Autodesk Inventor part; units mm, degrees
ref_plane "YZ Plane" through (0, 0, 0) normal (1, 0, 0) x (0, 1, 0)
ref_plane "XZ Plane" through (0, 0, 0) normal (0, 1, 0) x (-1, 0, 0)
ref_plane "XY Plane" through (0, 0, 0) normal (0, 0, 1) x (1, 0, 0)
sketch "Sketch1" plane through (0, 0, 0) normal (0, 0, 1) x (1, 0, 0)
  line L0 (0, 0) -> (53, 0)
  line L1 (53, 0) -> (53, -50)
  line L2 (53, -50) -> (0, -50)
  line L3 (0, -50) -> (0, 0)
  line L4 (41, 0) -> (41, 6.0159) construction
  line L5 (41, 6.0159) -> (41, -25.0024) construction
  circle A0 centre (41, -5) radius 1.5
  line L6 (41, 3.3654) -> (9, 3.3654) construction
  line L7 (9, 3.3654) -> (9, -23.8563) construction
  line L8 (41, -5) -> (7.1054, -5) construction
  circle A1 centre (9, -5) radius 1.5
  dimension "d0" = 53
  dimension "d1" = 50
  dimension "d2" = 3
  dimension "d3" = 32
  dimension "d4" = 3
extrude "Extrusion1" add sketch "Sketch1" along normal blind 3
sketch "Sketch2" plane through (0, 0, 3) normal (0, 0, 1) x (1, 0, 0)
  line L0 (53, -50) -> (15, -50)
  line L1 (15, -50) -> (15, -47)
  line L2 (15, -47) -> (53, -47)
  line L3 (53, -47) -> (53, -50)
  dimension "d7" = 38
  dimension "d8" = 3
extrude "Extrusion2" add sketch "Sketch2" against normal blind 12
fillet "Fillet3" radius 2 1 edges at (53, -48.5, -9)
fillet "Fillet6" radius 2 1 edges at (15, -48.5, -9)
sketch "Sketch5" plane through (0, 0, 3) normal (0, 0, 1) x (1, 0, 0)
  line L0 (18.1552, -8.3715) -> (42.9873, -8.3715)
  line L1 (42.9873, -8.3715) -> (42.9873, -35.5989)
  line L2 (42.9873, -35.5989) -> (18.1552, -35.5989)
  line L3 (18.1552, -35.5989) -> (18.1552, -8.3715)
extrude "Extrusion4" cut sketch "Sketch5" against normal through all
fillet "Fillet8" radius 2 1 edges at (18.1552, -8.3715, 1.5)
fillet "Fillet9" radius 2 1 edges at (42.9873, -8.3715, 1.5)
fillet "Fillet10" radius 2 1 edges at (18.1552, -35.5989, 1.5)
fillet "Fillet12" radius 2 1 edges at (42.9873, -35.5989, 1.5)
fillet "Fillet13" radius 2 1 edges at (0, 0, 1.5)
fillet "Fillet14" radius 2 1 edges at (53, 0, 1.5)
hole "Hole3" at (17.1081, -4.4429, 3) direction (0, 0, -1) diameter 3 end through all
sketch "Sketch6" plane through (0, -50, 3) normal (0, -1, 0) x (1, 0, 0)
  line L0 (51, -12) -> (17, -12)
  line L1 (0, 0) -> (53, 0)
  line L2 (53, 0) -> (51, 0) construction
  line L3 (51, 2) -> (51, -15) construction
  line L4 (54, -9) -> (12.4146, -9) construction
  line L5 (51, -7.4819) -> (20, -7.4819) construction
  line L6 (20, -7.4819) -> (20, -11) construction
  circle A0 centre (20, -9) radius 1.5
  circle A1 centre (51, -9) radius 1.5
  dimension "d60" = 31
  dimension "d61" = 3
  dimension "d64" = 3
extrude "Extrusion5" cut sketch "Sketch6" against normal through all contours A0
extrude "Extrusion6" cut sketch "Sketch6" against normal through all contours A1
sketch "Sketch7" plane through (0, 0, 3) normal (0, 0, 1) x (1, 0, 0)
  line L0 (40.9873, -35.5989) -> (20.1552, -35.5989)
  line L1 (0, -50) -> (53, -50)
  line L2 (32.5151, -35.5989) -> (24.407, -50)
  line L3 (40.0869, -35.5989) -> (47.0869, -50)
  point P0 (0, 0)
extrude "Extrusion7" cut sketch "Sketch7" against normal through all
sketch "Sketch8" plane through (0, 0, 3) normal (0, 0, 1) x (1, 0, 0)
  line L0 (0, -50) -> (24.407, -50)
  circle A0 centre (9, -5) radius 1.5
  line L1 (0, 0) -> (12, 0)
  line L2 (12, 0) -> (12, -50)
  line L3 (12, -50) -> (0, -50)
  line L4 (0, -50) -> (0, 0)
extrude "Extrusion8" cut sketch "Sketch8" against normal through all
fillet "Fillet15" radius 2 1 edges at (12, -50, 1.5)
fillet "Fillet16" radius 2 1 edges at (12, 0, 1.5)
properties part number "bart z endstop bracket v3"
For this review, take the finished solid that the model builds, in its own axes (mm). A direction names the side the tool comes from. Coordinates: 2 decimals unless noted, no trailing zeros. Write each loop counter-clockwise with the first axis right and the second up, starting at its lowest first coordinate (ties: lowest second). Pieces come first, ordered by that corner, then holes. Notation, with made-up numbers: (-9.75, 8.5) - (42.25, 8.5) arc R30 cw to (42.25, 43.5) - close; hole circle Ø10 at (-29, -9). An arc over 180 degrees is marked (long way). Answer in a Markdown table with one row per item. Add a question column.
Q1. We need section A-A, the plane z = -3.25. State the section outline as (x, y) points.
Q2. We need section C-C, the plane z = -6. State the section outline as (x, y) points, and give its area (3 significant figures).
Q3. For probe 1 along Z at (x, y) = (51, -48.5); probe 2 along Y at (x, z) = (41, 0.9); probe 3 along Y at (x, z) = (35, 2.25), list the stretches that pass through material, from the lowest coordinate up.
Q4. Tool access review of faces 4 (the flat face through (20, -47, -4)), 5 (the flat face through (30, -8.372, 2)), 6 (the flat face through (15, -49, -3)), 7 (the cylindrical face through (12.57, -0.6, 1.48)): name each direction out of +Z, -Z, +X, -X, +Y, -Y from which nothing blocks a thin tool from reaching the whole face with its end or side.
Q5. We need section D-D, the plane y = -5. State the section outline as (x, z) points.
Q6. Draft analysis for pull direction X (two halves, no side actions). For faces 1 (the flat face through (53, -29, 1)), 2 (the flat face through (26, -35.599, 2)), 3 (the flat face through (21, -48, -9)), state which applies: +X half, -X half, draft (parallel to the pull), parting line (faces both ways), or undercut.
Q7. For P1, Ø2, axis at x = 35.5, z = 1.5, coming from the +Y side; P2, Ø2.5, axis at x = 17.11, y = -4.44, coming from the -Z side; P3, Ø5, axis at x = 39.5, z = 1.5, coming from the -Y side; P4, Ø3.5, axis at y = -48.5, z = -4.5, coming from the -X side, all flat-tipped, find the tip position at first contact; note any pin that passes through.
Q8. We need section B-B, the plane y = -32. State the section outline as (x, z) points.
Answer list:
| question | item | result |
|---|---|---|
| 1 | outline | (15, -50) - (24.41, -50) - (26.1, -47) - (15, -47) - close; (45.63, -47) - (47.09, -50) - (53, -50) - (53, -47) - close |
| 2 | outline | (15, -50) - (18.5, -50) - (18.5, -47) - (15, -47) - close; (21.5, -50) - (24.41, -50) - (26.1, -47) - (21.5, -47) - close; (45.63, -47) - (47.09, -50) - (49.5, -50) - (49.5, -47) - close; (52.5, -50) - (53, -50) - (53, -47) - (52.5, -47) - close |
| 2 | area | 32.7 mm2 |
| 3 | probe 1 | z = -9 to -7.5, -4.5 to 3 |
| 3 | probe 2 | y = -37.48 to -35.6, -8.37 to -6.5, -3.5 to 0 |
| 3 | probe 3 | y = -8.37 to 0 |
| 4 | face 4 | -Z, +X, -X, +Y |
| 4 | face 5 | +Z, -Z |
| 4 | face 6 | -Z, -X, +Y, -Y |
| 4 | face 7 | +Z, -Z, -X, +Y |
| 5 | outline | (12, 0) - (15.72, 0) - (15.72, 3) - (12, 3) - close; (18.5, 0) - (39.5, 0) - (39.5, 3) - (18.5, 3) - close; (42.5, 0) - (53, 0) - (53, 3) - (42.5, 3) - close |
| 6 | face 1 | +X half |
| 6 | face 2 | undercut |
| 6 | face 3 | draft |
| 7 | P1 | stops at y = 0 |
| 7 | P2 | passes through |
| 7 | P3 | stops at y = -39.53 |
| 7 | P4 | stops at x = 15 |
| 8 | outline | (12, 0) - (18.16, 0) - (18.16, 3) - (12, 3) - close; (42.99, 0) - (53, 0) - (53, 3) - (42.99, 3) - close |
